Drawing for the job (mm, zero at the part's lowest x, y, z). Give positions to 0.01 mm unless a question says otherwise; leave off trailing zeros. Write each loop counter-clockwise with the first axis right and the second up, starting at its lowest first coordinate (ties: lowest second). Pieces come first, ordered by that corner, then holes. Notation, with made-up numbers: (46, -15.75) - (94, -15.75) arc R19 cw to (94, 16.25) - close; hole circle Ø5 at (9, 49). An arc over 180 degrees is marked (long way). Use CSV: the item, a comma, the result in double quotes.
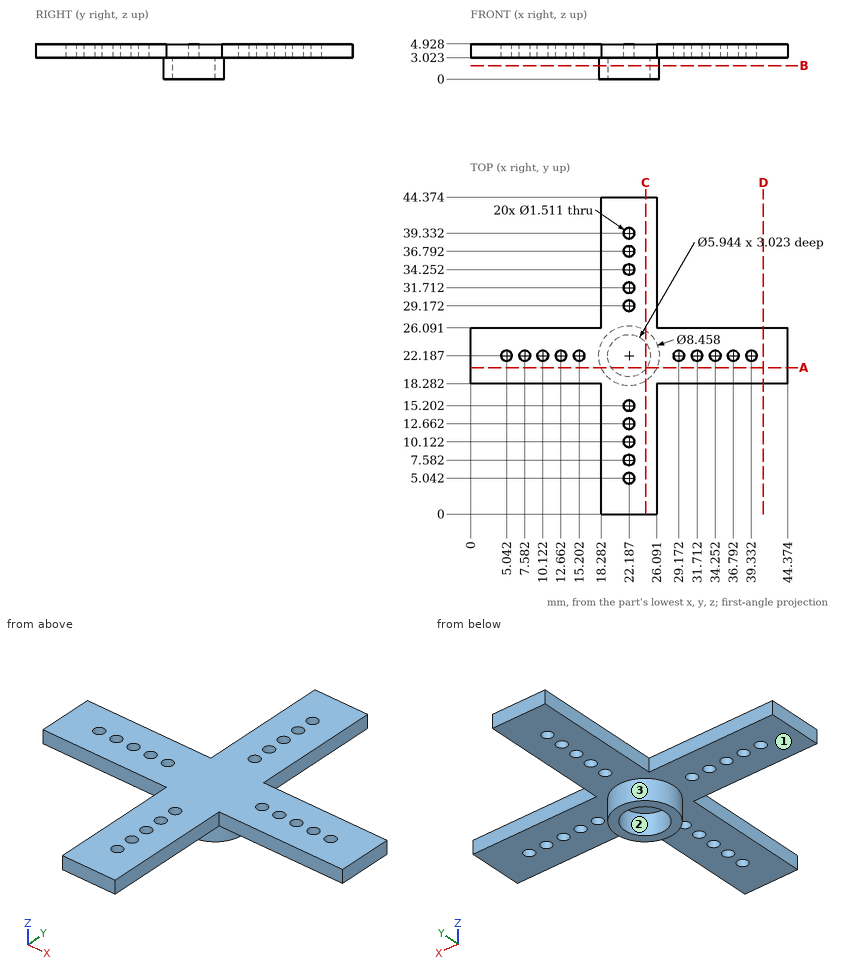
(1) Saw through at D-D, the plane x = 41. List the corners of the cut face in (y, z).
Checked values:
outline,"(18.28, 3.02) - (26.09, 3.02) - (26.09, 4.93) - (18.28, 4.93) - close"
(2) Flat gauge pins, fed straight in: P1, Ø1.5, axis at x = 34, z = 3, coming from the -Y side; P2, Ø2.5, axis at x = 36.79, y = 22.19, coming from the -Z side; P3, Ø0.9, axis at x = 5.04, y = 22.19, coming from the -Z side; P4, Ø1, axis at y = 10.5, z = 4, coming from the -X side. Where does each tip first touch, or does it go through?
Checked values:
P1,"stops at y = 18.28"
P2,"stops at z = 3.02"
P3,"passes through"
P4,"stops at x = 18.28"
(3) Saw through at A-A, the plane y = 20.5. List the corners of the cut face in (x, z) (1 decimal).
Checked values:
outline,"(0, 3) - (18.3, 3) - (18.3, 0) - (19.7, 0) - (19.7, 3) - (24.6, 3) - (24.6, 0) - (26.1, 0) - (26.1, 3) - (44.4, 3) - (44.4, 4.9) - (0, 4.9) - close"
(4) Saw through at C-C, the plane x = 24.5. List the corners of the cut face in (y, z).
Checked values:
outline,"(0, 3.02) - (18.65, 3.02) - (18.65, 0) - (20.32, 0) - (20.32, 3.02) - (24.05, 3.02) - (24.05, 0) - (25.73, 0) - (25.73, 3.02) - (44.37, 3.02) - (44.37, 4.93) - (0, 4.93) - close"
(5) Wall check: probe 1 along Y at (x, z) = (22, 1.5); probe 2 along Y at (x, z) = (5, 3.45); probe 3 along Z at (x, y) = (21.5, 33). Give the ranges that are in metal, low to high. Write a range as [from, to].
Checked values:
probe 1,"y = [17.96, 19.22], [25.15, 26.41]"
probe 2,"y = [18.28, 21.43], [22.94, 26.09]"
probe 3,"z = [3.02, 4.93]"
(6) Saw through at B-B, the plane z = 1.9. List the corners of the cut face in (x, y) (1 decimal).
Checked values:
outline,"circle Ø8.5 at (22.2, 22.2); hole circle Ø5.9 at (22.2, 22.2)"
(7) Pull direction X, two halves, no side cores. Call the marked faces 1, 2 and 3: released by +X, released by -X, zero draft, split by the parting line, or undercut.
Checked values:
face 1,"zero draft"
face 2,"undercut"
face 3,"split by the parting line"
